Can you work these out from the model? Positions are in its coordinate system, mm. Face numbers are marked on the shaded views. A direction names the side the tool comes from. Give positions to 0.01 mm unless a question says otherwise; leave off trailing zeros. Order: outer loops, then holes, each group sorted by start corner. A loop starts at its lowest first (then second) coordinate and runs counter-clockwise, first axis right, second up. Notation, with made-up numbers: (23, -8) - (42, -8) arc R27 ccw to (42, 31) - close; hole circle Ø8 at (38.5, -20). An arc over 180 degrees is marked (long way). Use one line per item in the form item = value. Start each with the question number.
1) We'd pull the mould along X, two halves only. Please class the marked faces 1, 2 and 3: released by +X, released by -X, zero draft, split by the parting line, or undercut.
2) Suppose I cut it at A-A, the plane y = 0. State how many separate pieces and enclosed holes the cut face has, and give its area (3 significant figures).
3) Which directions (+Z, -Z, +X, -X, +Y, -Y) give clear straight access to the entire face, cutting with the end or side of a thin tool? Please do the marked faces 4 and 5.
4) Please list where these lines run through material, in increasing order: probe 1 along Z at (x, y) = (-3, 5); probe 2 along Y at (x, z) = (6.5, 0.75); probe 3 along Y at (x, z) = (-0.5, 4.5).
5) For pin 1 (0.5 mm diameter, centred on x = 6, z = 2, fed in from -Y); pin 2 (0.5 mm diameter, centred on y = 5.5, z = 1, fed in from -X); pin 3 (1.7 mm diameter, centred on x = -6, z = 1, fed in from +Y); pin 4 (1.5 mm diameter, centred on x = 5, y = -9.5, fed in from +Z), each with a flat end and sliding along its axis, tell me the tip position at first contact or that it passes through.
6) Suppose I cut it at C-C, the plane z = 4.25. Write out the boundary of the cut face in (x, y), and give its area (3 significant figures).
```python
from build123d import *

# Parameters (mm, degrees)
BOSS_EXTRUDE1_DEPTH   = 3
F_1_0MM_DOWEL_HOLE1_D = 1
LPATTERN1_COUNT       = 4
LPATTERN1_PITCH       = 3
CIRPATTERN1_COUNT     = 4
CIRPATTERN1_COPY_1_D  = 1
CIRPATTERN1_COPY_2_D  = 1
CIRPATTERN1_COPY_3_D  = 1
CIRPATTERN1_COPY_4_D  = 1
CIRPATTERN1_COPY_5_D  = 1
CIRPATTERN1_COPY_6_D  = 1
CIRPATTERN1_COPY_7_D  = 1
CIRPATTERN1_COPY_8_D  = 1
CIRPATTERN1_COPY_9_D  = 1
SKETCH6_R             = 5
SKETCH6_R_2           = 3
BOSS_EXTRUDE2_DEPTH   = 3.5
CHAMFER1_SIZE         = 1
CHAMFER1_SIZE2        = 0.577350269
FILLET1_R             = 1


with BuildPart() as part:
    # Sketch1 → Boss-Extrude1 (new body)
    with BuildSketch(Plane.XY):
        with BuildLine():
            Line((-4, 0), (-4, 6.574293681))
            ThreePointArc((-4, 6.574293681), (-3.974394349, 6.996885575), (-3.897952052, 7.413294188))
            Line((-3.897952052, 7.413294188), (-1.698976026, 16.319147094))
            ThreePointArc((-1.698976026, 16.319147094), (0, 17.649646841), (1.698976026, 16.319147094))
            Line((1.698976026, 16.319147094), (3.897952052, 7.413294188))
            ThreePointArc((3.897952052, 7.413294188), (3.974394349, 6.996885575), (4, 6.574293681))
            Line((4, 6.574293681), (4, 0))
            Line((4, 0), (1.25, 0))
            ThreePointArc((1.25, 0), (0, 1.25), (-1.25, 0))
            Line((-1.25, 0), (-4, 0))
        make_face()
    boss_extrude1 = extrude(amount=BOSS_EXTRUDE1_DEPTH)

    # Ø1.0mm Dowel Hole1 (through all)
    with Locations(Plane.XY.offset(3)):
        with Locations((0, 15.899646841)):
            f_1_0mm_dowel_hole1 = Hole(F_1_0MM_DOWEL_HOLE1_D / 2)

    # LPattern1: Ø1.0mm Dowel Hole1 ×4
    with Locations(*[(0, -i * LPATTERN1_PITCH, 0) for i in range(1, LPATTERN1_COUNT)]):
        add(f_1_0mm_dowel_hole1, mode=Mode.SUBTRACT)

    # CirPattern1: Boss-Extrude1, Ø1.0mm Dowel Hole1 ×4 about axis
    cirpattern1_axis = Axis((0, 0, 0), (0, 0, 1))
    add([boss_extrude1.rotate(cirpattern1_axis, i * 360 / CIRPATTERN1_COUNT) for i in range(1, CIRPATTERN1_COUNT)])
    add([f_1_0mm_dowel_hole1.rotate(cirpattern1_axis, i * 360 / CIRPATTERN1_COUNT) for i in range(1, CIRPATTERN1_COUNT)], mode=Mode.SUBTRACT)

    # CirPattern1 copy 1 (through all)
    with Locations(Plane(origin=(3, 0, 3), x_dir=(0, 1, 0), z_dir=(0, 0, 1))):
        with Locations((0, 15.899646841)):
            Hole(CIRPATTERN1_COPY_1_D / 2)

    # CirPattern1 copy 2 (through all)
    with Locations(Plane(origin=(0, 3, 3), x_dir=(-1, 0, 0), z_dir=(0, 0, 1))):
        with Locations((0, 15.899646841)):
            Hole(CIRPATTERN1_COPY_2_D / 2)

    # CirPattern1 copy 3 (through all)
    with Locations(Plane(origin=(-3, 0, 3), x_dir=(0, -1, 0), z_dir=(0, 0, 1))):
        with Locations((0, 15.899646841)):
            Hole(CIRPATTERN1_COPY_3_D / 2)

    # CirPattern1 copy 4 (through all)
    with Locations(Plane(origin=(6, 0, 3), x_dir=(0, 1, 0), z_dir=(0, 0, 1))):
        with Locations((0, 15.899646841)):
            Hole(CIRPATTERN1_COPY_4_D / 2)

    # CirPattern1 copy 5 (through all)
    with Locations(Plane(origin=(0, 6, 3), x_dir=(-1, 0, 0), z_dir=(0, 0, 1))):
        with Locations((0, 15.899646841)):
            Hole(CIRPATTERN1_COPY_5_D / 2)

    # CirPattern1 copy 6 (through all)
    with Locations(Plane(origin=(-6, 0, 3), x_dir=(0, -1, 0), z_dir=(0, 0, 1))):
        with Locations((0, 15.899646841)):
            Hole(CIRPATTERN1_COPY_6_D / 2)

    # CirPattern1 copy 7 (through all)
    with Locations(Plane(origin=(9, 0, 3), x_dir=(0, 1, 0), z_dir=(0, 0, 1))):
        with Locations((0, 15.899646841)):
            Hole(CIRPATTERN1_COPY_7_D / 2)

    # CirPattern1 copy 8 (through all)
    with Locations(Plane(origin=(0, 9, 3), x_dir=(-1, 0, 0), z_dir=(0, 0, 1))):
        with Locations((0, 15.899646841)):
            Hole(CIRPATTERN1_COPY_8_D / 2)

    # CirPattern1 copy 9 (through all)
    with Locations(Plane(origin=(-9, 0, 3), x_dir=(0, -1, 0), z_dir=(0, 0, 1))):
        with Locations((0, 15.899646841)):
            Hole(CIRPATTERN1_COPY_9_D / 2)

    # Sketch6 → Boss-Extrude2 (add)
    with BuildSketch(Plane.XY.offset(3)):
        Circle(SKETCH6_R)
        Circle(SKETCH6_R_2, mode=Mode.SUBTRACT)
    extrude(amount=BOSS_EXTRUDE2_DEPTH)

    # Chamfer1
    chamfer1_edges = [part.edges().sort_by_distance(p)[0] for p in [
        (-5, 0, 6.5),
    ]]
    chamfer1_side = [part.faces().sort_by_distance(p)[0] for p in [
        (-5, 0, 4.75),
    ]]
    chamfer(chamfer1_edges, length=CHAMFER1_SIZE, length2=CHAMFER1_SIZE2, reference=chamfer1_side[0])

    # Fillet1
    fillet1_edges = [part.edges().sort_by_distance(p)[0] for p in [
        (4, 4, 1.5),
        (-4, 4, 1.5),
        (-4, -4, 1.5),
        (4, -4, 1.5),
    ]]
    fillet(fillet1_edges, radius=FILLET1_R)


solid = part.part
```
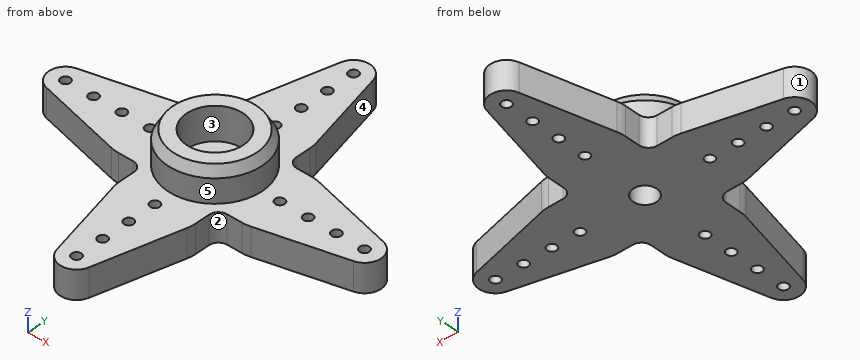
Result sheet:
q1.face_1 = released by -X
q1.face_2 = released by +X
q1.face_3 = undercut
q2.separate_pieces = 10
q2.enclosed_holes = 0
q2.area = 87.8 mm²
q3.face_4 = +Z, -Z, +X, +Y
q3.face_5 = +Z
q4.probe_1 = 0 to 3
q4.probe_2 = -4 to -0.3, 0.3 to 4
q4.probe_3 = -4.97 to -2.96, 2.96 to 4.97
q5.pin_1 = -4
q5.pin_2 = -4
q5.pin_3 = 4
q5.pin_4 = through
q6.outline = circle Ø10 at (0, 0); hole circle Ø6 at (0, 0)
q6.area = 50.3 mm²
